Geometry: see drawing. Coordinates: mm, zero at the bounding-box minimum. A direction names the side the tool comes from. Coordinates: 2 decimals unless noted, no trailing zeros. Loops run counter-clockwise (first coordinate to the right, second up) from the corner with the lowest first, then second, coordinate; pieces in that order, holes last.
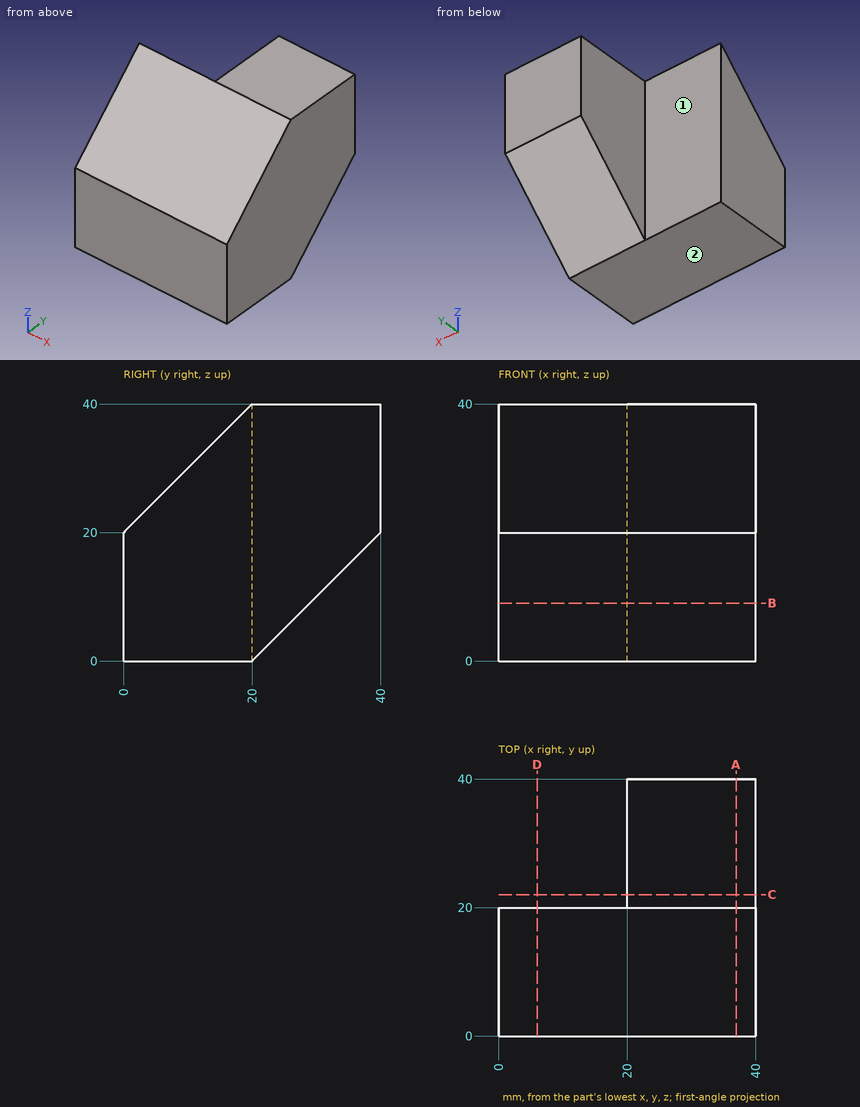
Item 1: Section query D-D (x = 6). Output: boundary loops of the cut face in (y, z).
Result:
outline: (0, 0) - (20, 0) - (20, 40) - (0, 20) - close
Item 2: Section query C-C (y = 22). Output: boundary loops of the cut face in (x, z), then the cut area to 3 significant figures.
Result:
outline: (20, 2) - (40, 2) - (40, 40) - (20, 40) - close
area: 760 mm2
Item 3: Section query A-A (x = 37). Output: boundary loops of the cut face in (y, z), then the cut area to 3 significant figures.
Result:
outline: (0, 0) - (20, 0) - (40, 20) - (40, 40) - (20, 40) - (0, 20) - close
area: 1,200 mm2
Item 4: Reachability of the marked faces 1 and 2 from +Z, -Z, +X, -X, +Y, -Y: full face, straight path, thin tool, end or side. Return the list, or none.
Result:
face 1: +Z, -Z, -X, +Y
face 2: -Z, +X, -X, +Y, -Y
Item 5: Contact query for flat-ended pins moving along their axis: P1, Ø4, axis at y = 9.5, z = 32.5, coming from the -X side; P2, Ø10, axis at x = 10.5, z = 22.5, coming from the +Y side; P3, Ø5, axis at x = 24.5, z = 23, coming from the -Y side; P4, Ø16, axis at y = 33, z = 21.5, coming from the -X side. Output: stop coordinate, or through.
Result:
P1: passes through
P2: stops at y = 20
P3: stops at y = 0.5
P4: stops at x = 20
Item 6: Line query: L1, parallel to X at y = 25.5, z = 38.5; L2, parallel to Y at x = 19, z = 13; L3, parallel to Z at x = 25, y = 9. Output: solid intervals per line, ascending.
Result:
L1: x = 20 to 40
L2: y = 0 to 20
L3: z = 0 to 29
Item 7: Section query B-B (z = 9). Output: boundary loops of the cut face in (x, y).
Result:
outline: (0, 0) - (40, 0) - (40, 29) - (20, 29) - (20, 20) - (0, 20) - close
